```python
from build123d import *

# Parameters (mm, degrees)
SKETCH_1_W      = 36
SKETCH_1_H      = 40
SKETCH_1_R      = 1.5
EXTRUDE_1_DEPTH = 4
SKETCH_13_W     = 4
SKETCH_13_H     = 40
EXTRUDE_2_DEPTH = 25


with BuildPart() as part:
    # Эскиз1 → Бобышка-Вытянуть1 (new body)
    with BuildSketch(Plane.XY):
        with Locations((18, 20)):
            Rectangle(SKETCH_1_W, SKETCH_1_H)
        with Locations((6, 30)):
            Circle(SKETCH_1_R, mode=Mode.SUBTRACT)
        with Locations((26, 30)):
            Circle(SKETCH_1_R, mode=Mode.SUBTRACT)
        with Locations((26, 10)):
            Circle(SKETCH_1_R, mode=Mode.SUBTRACT)
        with Locations((6, 10)):
            Circle(SKETCH_1_R, mode=Mode.SUBTRACT)
    extrude(amount=EXTRUDE_1_DEPTH)

    # Эскиз13 → Бобышка-Вытянуть2 (add)
    with BuildSketch(Plane(origin=(36, 0, 0), x_dir=(0, 0, -1), z_dir=(1, 0, 0))):
        with Locations((1.8, 20)):
            Rectangle(SKETCH_13_W, SKETCH_13_H)
    extrude(amount=EXTRUDE_2_DEPTH)


solid = part.part
```
The model under review builds one solid part; all positions refer to its coordinate system, in mm. A direction names the side the tool comes from. Give positions to 0.01 mm unless a question says otherwise; leave off trailing zeros. Write each loop counter-clockwise with the first axis right and the second up, starting at its lowest first coordinate (ties: lowest second). Pieces come first, ordered by that corner, then holes. Notation, with made-up numbers: (45, 10.25) -> (75, 10.25) arc R25 cw to (75, 42.25) -> close; hole circle Ø5 at (70.25, -5). An arc over 180 degrees is marked (long way). Put each result on its own line as item: value.
(1) Tool access review of faces 1 (the flat face through (18, 20, 0)), 2 (the flat face through (48, 20, 0.2)), 3 (the flat face through (0, 20, 2)): name each direction out of +Z, -Z, +X, -X, +Y, -Y from which nothing blocks a thin tool from reaching the whole face with its end or side.
Results are:
face 1: -Z, -X, +Y, -Y
face 2: +Z, +X, +Y, -Y
face 3: +Z, -Z, -X, +Y, -Y
(2) To check wall thickness, follow probe 1 along Y at (x, z) = (6, 0.75); probe 2 along Z at (x, y) = (6.5, 33.5); probe 3 along X at (y, z) = (11, -0.75). State the ranges of each line that lie inside material, in increasing order. Write a range as from..to.
Results are:
probe 1: 0..8.5, 11.5..28.5, 31.5..40
probe 2: 0..4
probe 3: 36..61
(3) We need section A-A, the plane y = 30. Give the boundary of the cut face in (x, z), and give its area (3 significant figures).
Results are:
outline: (0, 0) -> (4.5, 0) -> (4.5, 4) -> (0, 4) -> close; (7.5, 0) -> (24.5, 0) -> (24.5, 4) -> (7.5, 4) -> close; (27.5, 0) -> (36, 0) -> (36, -3.8) -> (61, -3.8) -> (61, 0.2) -> (36, 0.2) -> (36, 4) -> (27.5, 4) -> close
area: 220 mm²
(4) We need section B-B, the plane z = 1.5. Give the boundary of the cut face in (x, y), and give its area (3 significant figures).
Results are:
outline: (0, 0) -> (36, 0) -> (36, 40) -> (0, 40) -> close; hole circle Ø3 at (6, 10); hole circle Ø3 at (6, 30); hole circle Ø3 at (26, 10); hole circle Ø3 at (26, 30)
area: 1,410 mm²
(5) We need section D-D, the plane y = 23.5. Give the boundary of the cut face in (x, z), and give its area (3 significant figures).
Results are:
outline: (0, 0) -> (36, 0) -> (36, -3.8) -> (61, -3.8) -> (61, 0.2) -> (36, 0.2) -> (36, 4) -> (0, 4) -> close
area: 244 mm²
(6) We need section C-C, the plane x = 6. Give the boundary of the cut face in (y, z).
Results are:
outline: (0, 0) -> (8.5, 0) -> (8.5, 4) -> (0, 4) -> close; (11.5, 0) -> (28.5, 0) -> (28.5, 4) -> (11.5, 4) -> close; (31.5, 0) -> (40, 0) -> (40, 4) -> (31.5, 4) -> close
(7) For pin 1 Ø3 at (y, z) = (19, 0.5) entering from +X; pin 2 Ø10 at (x, y) = (21.5, 9) entering from -Z; pin 3 Ø2 at (y, z) = (14.5, 2) entering from +X; pin 4 Ø12.5 at (x, y) = (53, 14.5) entering from +Z, all flat-tipped, find the tip position at first contact; note any pin that passes through.
Results are:
pin 1: x = 61
pin 2: z = 0
pin 3: x = 36
pin 4: z = 0.2
(8) The part is to be moulded in two halves that separate along Y. For faces 4 (the cylindrical face through (24.89, 31.01, 1.97)), 5 (the flat face through (30.1, 40, 0.2)), 6 (the flat face through (18, 20, 4)), say which applies: pulls with the +Y half, pulls with the -Y half, needs draft (parallel to the pull), parting line crosses it, or undercut.
Results are:
face 4: undercut
face 5: pulls with the +Y half
face 6: needs draft
